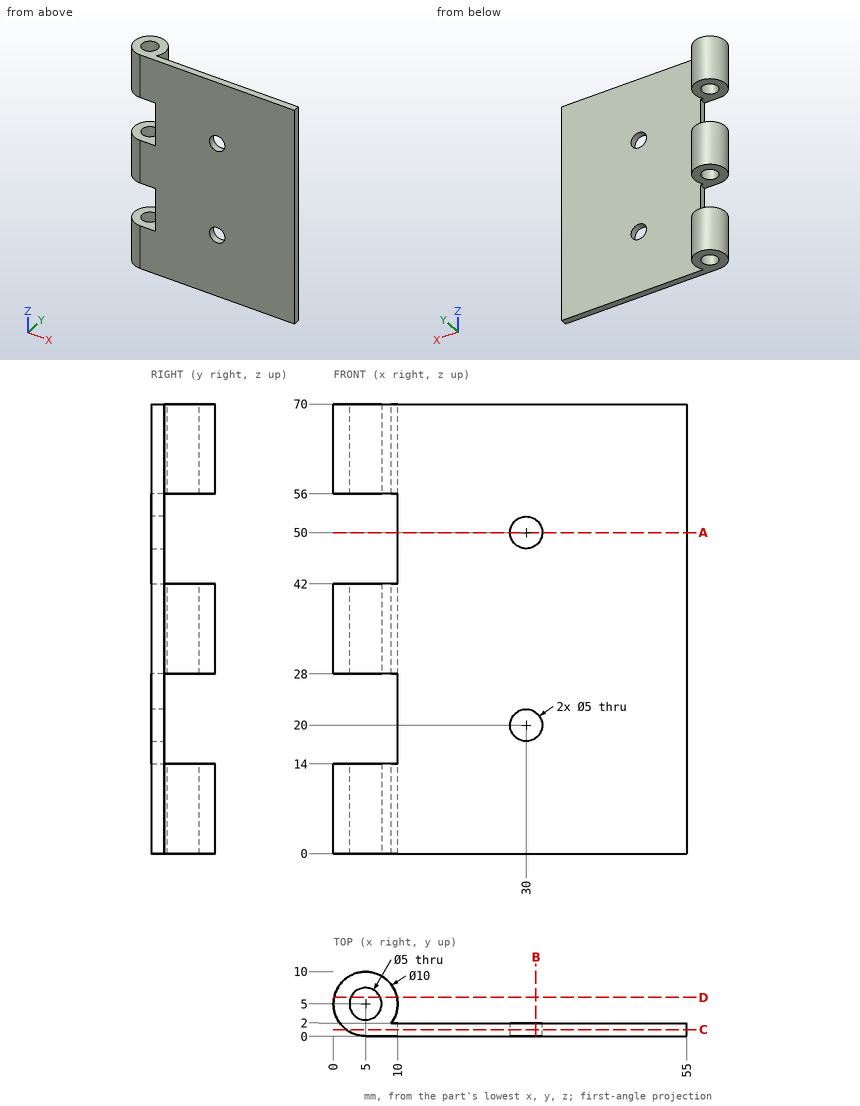
Print and shaded views of the part. All mm, measured from the part's lowest x, y and z. Coordinates: 2 decimals unless noted, no trailing zeros. Order: outer loops, then holes, each group sorted by start corner. A loop starts at its lowest first (then second) coordinate and runs counter-clockwise, first axis right, second up. Notation, with made-up numbers: M 23.25,56.5 L 51.25,56.5 A21 cw 51.25,72.5 Z; hole C 45,17 d5. An arc over 180 degrees is marked long. One line per question, with ' | ' between items. Start each with the question number.
Q1. Flat gauge pins, fed straight in: pin 1 Ø5 at (y, z) = (5, 37.5) entering from +X; pin 2 Ø0.6 at (y, z) = (1, 20) entering from -X; pin 3 Ø5 at (x, z) = (38.5, 8) entering from +Y. Where does each tip first touch, or does it go through?
Q2. Saw through at A-A (z = 50). List the corners of the cut face in (x, y).
Q3. Saw through at D-D (y = 6). List the corners of the cut face in (x, z).
Q4. Probe L1, parallel to Z at x = 2.5, y = 1.5; L2, parallel to Y at x = 5, z = 10.5; L3, parallel to X at y = 0.65, z = 50. List the from-to ranges inside material, lowest first. Write a range as from..to.
Q5. Saw through at C-C (y = 1). List the corners of the cut face in (x, z), then the cut area to 3 significant figures.
Q6. Saw through at B-B (x = 31.5). List the corners of the cut face in (y, z).
Check values:
1) pin 1: stops at x = 10 | pin 2: stops at x = 10 | pin 3: stops at y = 2
2) outline: M 10,0 L 27.5,0 L 27.5,2 L 10,2 Z; M 32.5,0 L 55,0 L 55,2 L 32.5,2 Z
3) outline: M 0.1,0 L 2.71,0 L 2.71,14 L 0.1,14 Z; M 0.1,28 L 2.71,28 L 2.71,42 L 0.1,42 Z; M 0.1,56 L 2.71,56 L 2.71,70 L 0.1,70 Z; M 7.29,0 L 9.9,0 L 9.9,14 L 7.29,14 Z; M 7.29,28 L 9.9,28 L 9.9,42 L 7.29,42 Z; M 7.29,56 L 9.9,56 L 9.9,70 L 7.29,70 Z
4) L1: z = 0..14, 28..42, 56..70 | L2: y = 0..2.5, 7.5..10 | L3: x = 10..27.5, 32.5..55
5) outline: M 2,0 L 55,0 L 55,70 L 2,70 L 2,56 L 10,56 L 10,42 L 2,42 L 2,28 L 10,28 L 10,14 L 2,14 Z; hole C 30,20 d5; hole C 30,50 d5 | area: 3,450 mm2
6) outline: M 0,0 L 2,0 L 2,18 L 0,18 Z; M 0,22 L 2,22 L 2,48 L 0,48 Z; M 0,52 L 2,52 L 2,70 L 0,70 Z
